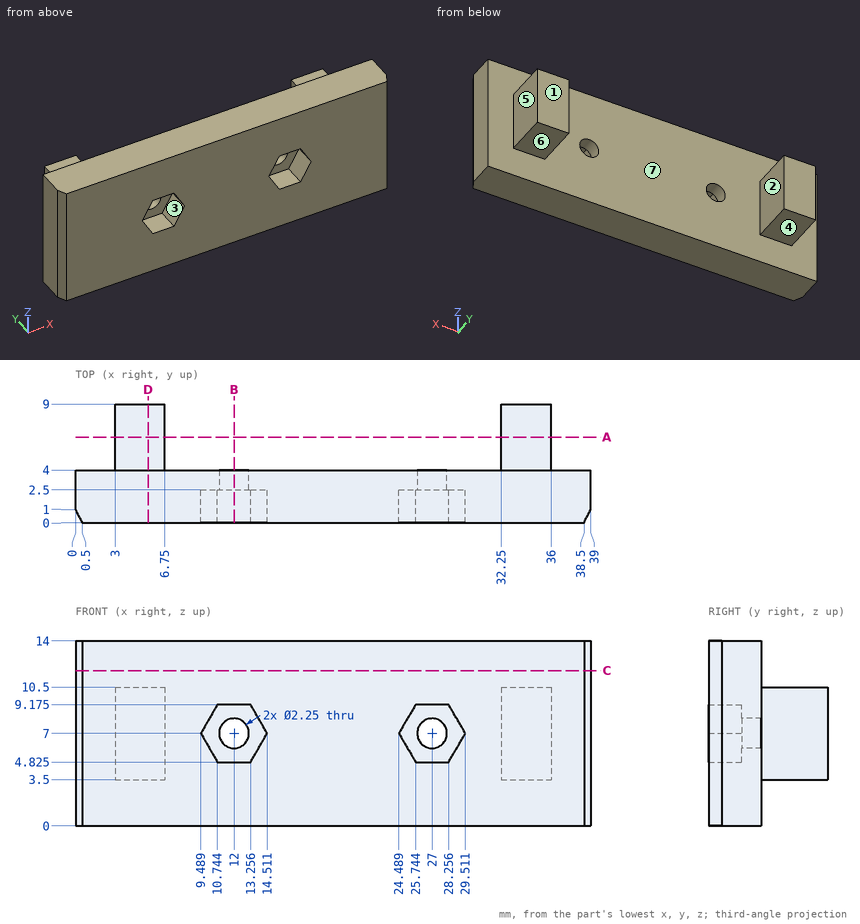
Print and shaded views of the part. All mm, measured from the part's lowest x, y and z. A direction names the side the tool comes from. Coordinates: 2 decimals unless noted, no trailing zeros. Order: outer loops, then holes, each group sorted by start corner. A loop starts at its lowest first (then second) coordinate and runs counter-clockwise, first axis right, second up. Notation, with made-up numbers: (81.25, 71) - (87.25, 71) arc R28 cw to (87.25, 92) - close; hole circle Ø1 at (86.5, -18.75). An arc over 180 degrees is marked (long way). Return JSON: item names as keys, results as strings. Group by question number.
Item 1: Which spindle directions (+Z, -Z, +X, -X, +Y, -Y) get a long thin tool onto all of the face, cutting with end or side? Do the marked faces 1, 2, 3 and 4. Say none if no direction does.
Item 2: Pull direction X, two halves, no side cores. Call the marked faces 5, 6 and 7: pulls with the +X half, pulls with the -X half, needs draft (parallel to the pull), parting line crosses it, or undercut.
Item 3: Cut at B-B (x = 12). List the corners of the cut face in (y, z) (1 decimal).
Item 4: Cut at C-C (z = 11.75). List the corners of the cut face in (x, y).
Item 5: Cut at D-D (x = 5.5). List the corners of the cut face in (y, z).
Item 6: Drill centre lines: probe 1 along X at (y, z) = (6.5, 7.5); probe 2 along Z at (x, y) = (12, 3.2) (1 decimal); probe 3 along Y at (x, z) = (10, 8.25). Where is each one in solid material? Low to high. Write a range as from..to.
Item 7: Pin check, flat tips, straight feed: pin 1 (2 mm diameter, centred on x = 13.5, z = 8.5, fed in from +Y); pin 2 (1 mm diameter, centred on y = 5, z = 4, fed in from +X); pin 3 (1 mm diameter, centred on x = 27, y = 5, fed in from -Z); pin 4 (4 mm diameter, centred on x = 35, y = 7.5, fed in from +Z). Stop position of each tip, or through.
Item 8: Cut at A-A (y = 6.5). List the corners of the cut face in (x, z).
Check values:
{
 "1": {"face 1": "+Z, -Z, +X, -X, +Y", "face 2": "+Z, -Z, +Y", "face 3": "-Y", "face 4": "-Z, +X, -X, +Y"},
 "2": {"face 5": "pulls with the +X half", "face 6": "needs draft", "face 7": "undercut"},
 "3": {"outline": "(0, 0) - (4, 0) - (4, 5.9) - (2.5, 5.9) - (2.5, 4.8) - (0, 4.8) - close; (0, 9.2) - (2.5, 9.2) - (2.5, 8.1) - (4, 8.1) - (4, 14) - (0, 14) - close"},
 "4": {"outline": "(0, 1) - (0.5, 0) - (38.5, 0) - (39, 1) - (39, 4) - (0, 4) - close"},
 "5": {"outline": "(0, 0) - (4, 0) - (4, 3.5) - (9, 3.5) - (9, 10.5) - (4, 10.5) - (4, 14) - (0, 14) - close"},
 "6": {"probe 1": "x = 3..6.75, 32.25..36", "probe 2": "z = 0..5.9, 8.1..14", "probe 3": "y = 0..4"},
 "7": {"pin 1": "stops at y = 4", "pin 2": "stops at x = 36", "pin 3": "passes through", "pin 4": "stops at z = 10.5"},
 "8": {"outline": "(3, 3.5) - (6.75, 3.5) - (6.75, 10.5) - (3, 10.5) - close; (32.25, 3.5) - (36, 3.5) - (36, 10.5) - (32.25, 10.5) - close"}
}
